Could you check a few things on this drawing? It's one solid part, dimensions in mm from its lowest x, y, z. Give positions to 0.01 mm unless a question says otherwise; leave off trailing zeros. Order: outer loops, then holes, each group sorted by start corner. A loop starts at its lowest first (then second) coordinate and runs counter-clockwise, first axis right, second up.
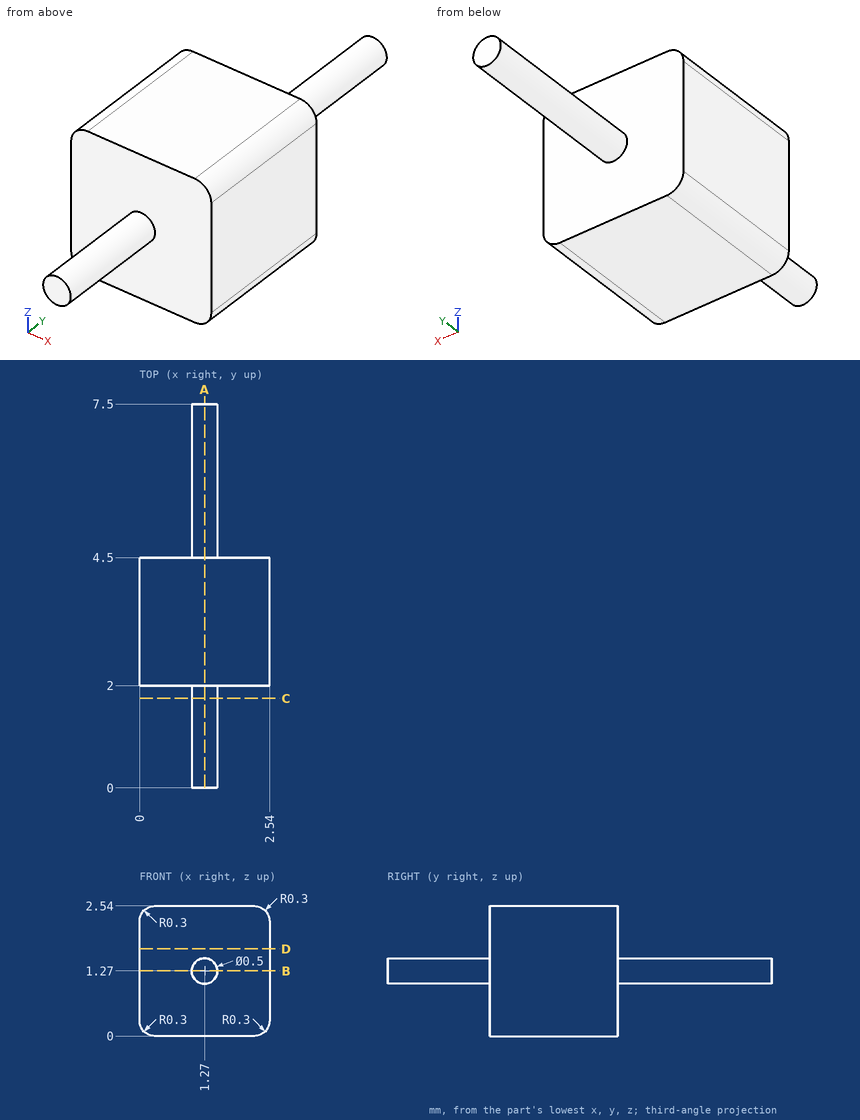
Item 1: Please list where these lines run through material, in increasing order: line 1 along Y through (x, z) = (0.5, 0.1); line 2 along Z through (x, y) = (1.3, 1); line 3 along Z through (x, y) = (0.2, 3.75).
Findings:
line 1: y = 2 to 4.5
line 2: z = 1.02 to 1.52
line 3: z = 0.02 to 2.52
Item 2: Imagine slicing it at C-C on y = 1.75. List the corners of the cut face in (x, z) for me, then the cut area to 3 significant figures.
Findings:
outline: circle Ø0.5 at (1.27, 1.27)
area: 0.196 mm2
Item 3: Imagine slicing it at B-B on z = 1.27. List the corners of the cut face in (x, y) for me, then the cut area to 3 significant figures.
Findings:
outline: (0, 2) - (1.02, 2) - (1.02, 0) - (1.52, 0) - (1.52, 2) - (2.54, 2) - (2.54, 4.5) - (1.52, 4.5) - (1.52, 7.5) - (1.02, 7.5) - (1.02, 4.5) - (0, 4.5) - close
area: 8.85 mm2
Item 4: For pin 1 (1 mm diameter, centred on x = 2, z = 0.5, fed in from +Y), with a flat end and sliding along its axis, tell me the tip position at first contact or that it passes through.
Findings:
pin 1: stops at y = 4.5
Item 5: Imagine slicing it at A-A on x = 1.27. List the corners of the cut face in (y, z) for me.
Findings:
outline: (0, 1.02) - (2, 1.02) - (2, 0) - (4.5, 0) - (4.5, 1.02) - (7.5, 1.02) - (7.5, 1.52) - (4.5, 1.52) - (4.5, 2.54) - (2, 2.54) - (2, 1.52) - (0, 1.52) - close
Item 6: Imagine slicing it at D-D on z = 1.7. List the corners of the cut face in (x, y) for me.
Findings:
outline: (0, 2) - (2.54, 2) - (2.54, 4.5) - (0, 4.5) - close
